```python
from build123d import *

# Parameters (mm, degrees)
F_8_CLEARANCE_HOLE1_D     = 4.4958
F_8_CLEARANCE_HOLE1_DEPTH = 3.176
CIRPATTERN1_COUNT         = 6
SKETCH4_R                 = 88.9
CUT_EXTRUDE1_DEPTH        = 13.7
BOSS_EXTRUDE2_START       = 0.254
SKETCH5_R                 = 88.9
BOSS_EXTRUDE2_DEPTH       = 2.54


with BuildPart() as part:
    # Sketch1 → Revolve1 (revolve)
    with BuildSketch(Plane(origin=(0, 0, 0), x_dir=(0, 0, -1), z_dir=(1, 0, 0))):
        Polygon((89.535, 0), (92.71, 0), (92.71, 9.525), (124.46, 9.525), (124.46, 12.7), (0, 12.7), (0, 9.525), (89.535, 9.525), align=None)
    revolve(axis=Axis((0, 0, 0), (0, 1, 0)))

    # #8 Clearance Hole1
    with Locations(Plane(origin=(0, 12.7, 0), x_dir=(1, 0, 0), z_dir=(0, 1, 0))):
        with Locations((0, 114.3)):
            f_8_clearance_hole1 = Hole(F_8_CLEARANCE_HOLE1_D / 2, depth=F_8_CLEARANCE_HOLE1_DEPTH)

    # CirPattern1: #8 Clearance Hole1 ×6 about axis
    cirpattern1_axis = Axis((0, 0, 0), (0, 1, 0))
    for i in range(1, CIRPATTERN1_COUNT):
        add(f_8_clearance_hole1.rotate(cirpattern1_axis, i * 360 / CIRPATTERN1_COUNT), mode=Mode.SUBTRACT)

    # Sketch4 → Cut-Extrude1 (cut, through all)
    with BuildSketch(Plane(origin=(0, 12.7, 0), x_dir=(1, 0, 0), z_dir=(0, 1, 0))):
        Circle(SKETCH4_R)
    extrude(amount=-CUT_EXTRUDE1_DEPTH, mode=Mode.SUBTRACT)

    # Sketch5 → Boss-Extrude2 (add)
    with BuildSketch(Plane(origin=(0, 12.7, 0), x_dir=(1, 0, 0), z_dir=(0, 1, 0)).offset(BOSS_EXTRUDE2_START)):
        Circle(SKETCH5_R)
    extrude(amount=-BOSS_EXTRUDE2_DEPTH)


solid = part.part
```
For this review, take the finished solid that the model builds, in its own axes (mm). A direction names the side the tool comes from. Coordinates: 2 decimals unless noted, no trailing zeros. Order: outer loops, then holes, each group sorted by start corner. A loop starts at its lowest first (then second) coordinate and runs counter-clockwise, first axis right, second up. Notation, with made-up numbers: (8.25, 33.5) - (28.25, 33.5) arc R21 ccw to (28.25, 66.5) - close; hole circle Ø4 at (-29.5, 51.25). An arc over 180 degrees is marked (long way). Answer as a JSON object with one key per item and string values. Group by question number.
1. Clearance check with flat-ended pins moving along their axes: P1, Ø1, axis at x = -96, z = -52.5, coming from the +Y side; P2, Ø3.5, axis at x = -98.99, z = -57.15, coming from the -Y side; P3, Ø6, axis at y = 6, z = 6.5, coming from the -X side; P4, Ø5, axis at x = 98.99, z = -57.15, coming from the -Y side (3 decimals). State where each tip first meets the part, or that it passes through.
2. For probe 1 along Z at (x, y) = (0, 9.8); probe 2 along Z at (x, y) = (0, 10.85); probe 3 along X at (y, z) = (11.6, -57.15), list the stretches that pass through material, from the lowest coordinate up.
3. We need section D-D on z = -103.5. State the section outline as (x, y) points (3 decimals).
4. The part is to be moulded in two halves that separate along X. For faces 1 (the flat face through (-29, 12.7, 85)), 2 (the cylindrical face through (35.51, 4.83, -85.64)), 3 (the cylindrical face through (-26.9, 4.7, -85.4)), say which applies: pulls with the +X half, pulls with the -X half, needs draft (parallel to the pull), parting line crosses it, or undercut.
5. For faces 4 (the flat face through (-93, 9.525, 9)), 5 (the cylindrical face through (121.5, 11.13, 26.98)), list the 3-axis set-ups (+Z, -Z, +X, -X, +Y, -Y) from which the entire face can be reached by the end or side of a thin tool; tool diameter is ignored.
6. We need section A-A on y = 3. State the section outline as (x, z) points (3 decimals), then the cut area to 3 significant figures.
Final values:
{
 "1": {"P1": "y = 12.7", "P2": "through", "P3": "x = -92.64", "P4": "y = 9.525"},
 "2": {"probe 1": "-124.46 to -116.55, -112.05 to -88.9, 88.9 to 112.05, 116.55 to 124.46", "probe 2": "-124.46 to -116.55, -112.05 to 112.05, 116.55 to 124.46", "probe 3": "-110.56 to -101.23, -96.74 to 96.74, 101.23 to 110.56"},
 "3": {"outline": "(-69.123, 9.525) - (69.123, 9.525) - (69.123, 12.7) - (-69.123, 12.7) - close"},
 "4": {"face 1": "needs draft", "face 2": "parting line crosses it", "face 3": "undercut"},
 "5": {"face 4": "-Y", "face 5": "+Y, -Y"},
 "6": {"outline": "circle Ø185.42 at (0, 0); hole circle Ø179.07 at (0, 0)", "area": "1,820 mm²"}
}
